Here's how the part is built. I have some questions about the finished solid (model axes, mm). Face numbers are marked on the shaded views. A direction names the side the tool comes from. Give positions to 0.01 mm unless a question says otherwise; leave off trailing zeros. Loops run counter-clockwise (first coordinate to the right, second up) from the corner with the lowest first, then second, coordinate; pieces in that order, holes last.
Q1. For the marked faces 1 and 2, which set-ups out of +Z, -Z, +X, -X, +Y, -Y let a thin tool reach every point of the face, with its end or its side?
Q2. Thinking about a two-plate mould opening in X: for the marked faces 3, 4, 5 and 6, which applies, pulls with the +X half, pulls with the -X half, needs draft (parallel to the pull), parting line crosses it, or undercut?
Q3. I'm going to push flat-ended pins straight in: P1, Ø4, axis at x = -24, y = -40.5, coming from the +Z side; P2, Ø0.6, axis at x = 12.5, z = 68.5, coming from the -Y side; P3, Ø2, axis at y = -45, z = 68.5, coming from the +X side; P4, Ø5.5, axis at x = 13.5, y = -43, coming from the +Z side. Where does each tip first touch, or does it pass through?
Q4. Suppose I cut it at A-A (y = -27.5). List the corners of the cut face in (x, z) for me.
Q5. I need wall thicknesses on probe 1 along X at (y, z) = (-66, 30); probe 2 along Z at (x, y) = (13, -19); probe 3 along X at (y, z) = (-49, 43). Which ranges of each line are inside material? Lowest first, please.
```python
from build123d import *

# Parameters (mm, degrees)
F0_W         = 85.2558612823
F0_H         = 85.4500681162
F1_DEPTH     = 82
F3_D         = 75
F3_DEPTH     = 60
F3_TIP       = 22.5322732135
F4_R         = 10
F5_R         = 10
F6_R         = 10
F7_R         = 10
F8_T1_DEPTH  = 62
F8_T3_DEPTH  = 65.2558612823
F8_T5_DEPTH  = 65.4500681162
F8_S9_W      = 10
F8_S9_H      = 10
F8_T10_DEPTH = 10
F8_S15_W     = 10
F8_S15_H     = 10
F8_T16_DEPTH = 10
F8_T20_ANGLE = 90
F8_T22_ANGLE = 90
F8_T24_ANGLE = 90
F9_W         = 26.7179913353
F9_H         = 11.2215578556
F10_DEPTH    = 2


# Not quite as in the source:
# - a fillet or chamfer that OpenCascade refuses, or shapes differently, is made with other operations: its cross-section is extruded or revolved along the edge and cut away or added


with BuildPart() as f1:
    # F0 (on Front) → F1 (new body)
    with BuildSketch(Plane.XZ):
        with Locations((9.4189271331, 27.0915552974)):
            Rectangle(F0_W, F0_H)
    extrude(amount=F1_DEPTH)

    # F3
    with Locations(Plane.XZ.offset(82)):
        with Locations((8.7392125279, 29.616214335)):
            Hole(F3_D / 2, depth=F3_DEPTH)
            with Locations((0, 0, -(F3_DEPTH + F3_TIP / 2))):  # 118° drill point
                Cone(0, F3_D / 2, F3_TIP, mode=Mode.SUBTRACT)

    # F4
    f4_edges = [f1.edges().sort_by_distance(p)[0] for p in [
        (52.046858, -41, 69.816589),
    ]]
    fillet(f4_edges, radius=F4_R)

    # F5
    f5_edges = [f1.edges().sort_by_distance(p)[0] for p in [
        (-33.209004, -41, 69.816589),
    ]]
    fillet(f5_edges, radius=F5_R)

    # F6
    f6_edges = [f1.edges().sort_by_distance(p)[0] for p in [
        (52.046858, -41, -15.633479),
    ]]
    fillet(f6_edges, radius=F6_R)

    # F7
    f7_edges = [f1.edges().sort_by_distance(p)[0] for p in [
        (4.418927, 0, -15.633479),
    ]]
    fillet(f7_edges, radius=F7_R)

    # F8: fillet of radius 10 on 2 edges, made by hand

    # F8_s2 → F8_t1 (cut)
    with BuildSketch(Plane.XZ.offset(10)):
        with BuildLine():
            ThreePointArc((-23.2090035081, -15.6334787607), (-30.28007132, -12.7045465726), (-33.2090035081, -5.6334787607))
            Line((-33.2090035081, -5.6334787607), (-33.2090035081, -15.6334787607))
            Line((-33.2090035081, -15.6334787607), (-23.2090035081, -15.6334787607))
        make_face()
    extrude(amount=F8_T1_DEPTH, mode=Mode.SUBTRACT)

    # F8_s4 → F8_t3 (cut)
    with BuildSketch(Plane.YZ.offset(-23.2090035081)):
        with BuildLine():
            ThreePointArc((-72, 69.8165893555), (-79.0710678119, 66.8876571673), (-82, 59.8165893555))
            Line((-82, 59.8165893555), (-82, 69.8165893555))
            Line((-82, 69.8165893555), (-72, 69.8165893555))
        make_face()
        with BuildLine():
            ThreePointArc((-72, -15.6334787607), (-79.0710678119, -12.7045465726), (-82, -5.6334787607))
            Line((-82, -5.6334787607), (-82, -15.6334787607))
            Line((-82, -15.6334787607), (-72, -15.6334787607))
        make_face()
    extrude(amount=F8_T3_DEPTH, mode=Mode.SUBTRACT)

    # F8_s6 → F8_t5 (cut)
    with BuildSketch(Plane.XY.offset(-5.6334787607)):
        with BuildLine():
            ThreePointArc((-33.2090035081, -72), (-30.28007132, -79.0710678119), (-23.2090035081, -82))
            Line((-23.2090035081, -82), (-33.2090035081, -82))
            Line((-33.2090035081, -82), (-33.2090035081, -72))
        make_face()
        with BuildLine():
            ThreePointArc((52.0468577743, -72), (49.1179255861, -79.0710678119), (42.0468577743, -82))
            Line((42.0468577743, -82), (52.0468577743, -82))
            Line((52.0468577743, -82), (52.0468577743, -72))
        make_face()
    extrude(amount=F8_T5_DEPTH, mode=Mode.SUBTRACT)


with BuildPart() as f8_tool8:
    # F8_s9 → F8_t10 (new body)
    with BuildSketch(Plane.XY.offset(-5.6334787607)):
        with Locations((-28.2090035081, -5)):
            Rectangle(F8_S9_W, F8_S9_H)
    extrude(amount=-F8_T10_DEPTH)

    # F8_s11 → F8_t12 (revolve, cut)
    with BuildSketch(Plane(origin=(-23.2090035081, -10, -5.6334787607), x_dir=(0.7071067812, -0.7071067812, 0), z_dir=(0.7071067812, 0.7071067812, 0))):
        with BuildLine():
            ThreePointArc((0, -10), (10, 0), (0, 10))
            Line((0, 10), (0, -10))
        make_face()
    revolve(axis=Axis((-23.2090035081, -10, -5.6334787607), (0, 0, -1)), mode=Mode.SUBTRACT)


with BuildPart() as f1_1:
    add(f1.part)

    # F8_t7: cut F8_tool8
    add(f8_tool8.part, mode=Mode.SUBTRACT)


with BuildPart() as f8_tool14:
    # F8_s15 → F8_t16 (new body)
    with BuildSketch(Plane.YZ.offset(-23.2090035081)):
        with Locations((-77, -10.6334787607)):
            Rectangle(F8_S15_W, F8_S15_H)
    extrude(amount=-F8_T16_DEPTH)

    # F8_s17 → F8_t18 (revolve, cut)
    with BuildSketch(Plane(origin=(-23.2090035081, -72, -5.6334787607), x_dir=(0, 0.7071067812, 0.7071067812), z_dir=(0, -0.7071067812, 0.7071067812))):
        with BuildLine():
            ThreePointArc((0, -10), (10, 0), (0, 10))
            Line((0, 10), (0, -10))
        make_face()
    revolve(axis=Axis((-23.2090035081, -72, -5.6334787607), (-1, 0, 0)), mode=Mode.SUBTRACT)


with BuildPart() as f1_2:
    add(f1_1.part)

    # F8_t13: cut F8_tool14
    add(f8_tool14.part, mode=Mode.SUBTRACT)

    # F8_s19 → F8_t20 (revolve, cut)
    with BuildSketch(Plane.YZ.offset(42.0468577743)):
        with BuildLine():
            ThreePointArc((-82, 59.8165893555), (-79.0710678119, 66.8876571673), (-72, 69.8165893555))
            Line((-72, 69.8165893555), (-82, 69.8165893555))
            Line((-82, 69.8165893555), (-82, 59.8165893555))
        make_face()
    revolve(axis=Axis((42.0468577743, -82, 59.8165893555), (0, 1, 0)), revolution_arc=F8_T20_ANGLE, mode=Mode.SUBTRACT)

    # F8_s21 → F8_t22 (revolve, cut)
    with BuildSketch(Plane.YZ.offset(-23.2090035081)):
        with BuildLine():
            ThreePointArc((-82, 59.8165893555), (-79.0710678119, 66.8876571673), (-72, 69.8165893555))
            Line((-72, 69.8165893555), (-82, 69.8165893555))
            Line((-82, 69.8165893555), (-82, 59.8165893555))
        make_face()
    revolve(axis=Axis((-23.2090035081, -82, 59.8165893555), (0, -1, 0)), revolution_arc=F8_T22_ANGLE, mode=Mode.SUBTRACT)

    # F8_s23 → F8_t24 (revolve, cut)
    with BuildSketch(Plane.XY.offset(-5.6334787607)):
        with BuildLine():
            ThreePointArc((52.0468577743, -72), (49.1179255861, -79.0710678119), (42.0468577743, -82))
            Line((42.0468577743, -82), (52.0468577743, -82))
            Line((52.0468577743, -82), (52.0468577743, -72))
        make_face()
    revolve(axis=Axis((42.0468577743, -82, -5.6334787607), (0, 1, 0)), revolution_arc=F8_T24_ANGLE, mode=Mode.SUBTRACT)

    # F9 (on face) → F10 (cut)
    with BuildSketch(Plane.XY.offset(69.8165893555)):
        with Locations((9.8856553668, -43.1762188673)):
            Rectangle(F9_W, F9_H)
    extrude(amount=-F10_DEPTH, mode=Mode.SUBTRACT)


solid = f1_2.part
```
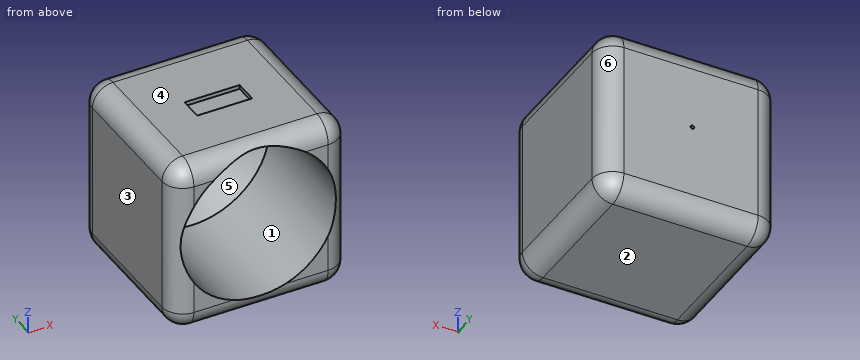
Solutions:
1. face 1: -Y
1. face 2: -Z, +X, -X, +Y, -Y
2. face 3: pulls with the -X half
2. face 4: needs draft
2. face 5: undercut
2. face 6: pulls with the +X half
3. P1: stops at z = 69.82
3. P2: stops at y = -77.45
3. P3: stops at x = 48.45
3. P4: stops at z = 67.82
4. outline: (-33.21, -5.63) arc R10 ccw to (-23.21, -15.63) - (42.05, -15.63) arc R10 ccw to (52.05, -5.63) - (52.05, 59.82) arc R10 ccw to (42.05, 69.82) - (-23.21, 69.82) arc R10 ccw to (-33.21, 59.82) - close; hole circle Ø75 at (8.74, 29.62)
5. probe 1: x = -33.21 to -28.76, 46.24 to 52.05
5. probe 2: z = -15.63 to -2.61, 61.84 to 69.82
5. probe 3: x = -33.21 to -26.29, 43.77 to 52.05
